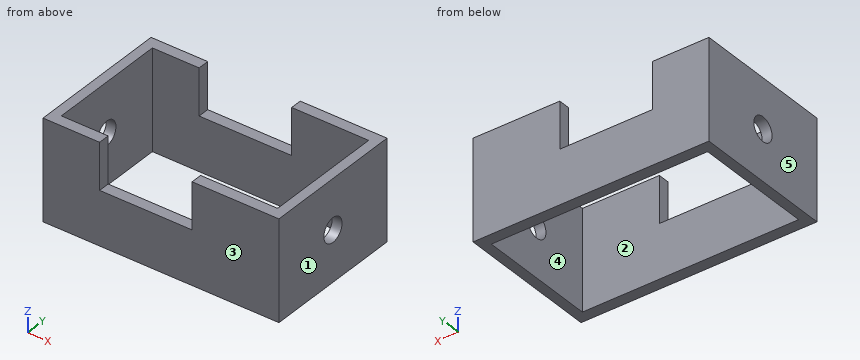
```python
from build123d import *

# Parameters (mm, degrees)
F0_W     = 170.937256
F0_H     = 103.51549
F1_DEPTH = 72.644
F2_W     = 156.719148
F2_H     = 87.184086
F3_DEPTH = 171.45
F4_W     = 67.018675
F4_H     = 33.684524
F6_DEPTH = 172.212
F7_R     = 8.715652
F8_DEPTH = 233.934


with BuildPart() as f1:
    # F0 (on Top) → F1 (new body)
    with BuildSketch(Plane.XY):
        Rectangle(F0_W, F0_H)
    extrude(amount=F1_DEPTH)

    # F2 (on face) → F3 (cut)
    with BuildSketch(Plane.XY.offset(72.644)):
        Rectangle(F2_W, F2_H)
    extrude(amount=-F3_DEPTH, mode=Mode.SUBTRACT)

    # F4 (on face) → F6 (cut)
    with BuildSketch(Plane.XZ.offset(51.757745)):
        with Locations((-10.945341, 55.801738)):
            Rectangle(F4_W, F4_H)
    extrude(amount=-F6_DEPTH, mode=Mode.SUBTRACT)

    # F7 (on face) → F8 (cut)
    with BuildSketch(Plane.YZ.offset(85.468628)):
        with Locations((0, 36.621507)):
            Circle(F7_R)
    extrude(amount=-F8_DEPTH, mode=Mode.SUBTRACT)


solid = f1.part
```
Input: part model. Units: mm. Frame: model coordinates. Face numbers are marked on the shaded views. A direction names the side the tool comes from. Round coordinates to 2 decimals unless told otherwise and drop trailing zeros. Order: outer loops, then holes, each group sorted by start corner. A loop starts at its lowest first (then second) coordinate and runs counter-clockwise, first axis right, second up. Notation, with made-up numbers: (-16, -16.5) - (17, -16.5) arc R15 ccw to (17, 9.5) - close; hole circle Ø11 at (75.25, -5). An arc over 180 degrees is marked (long way). One line per question, with ' | ' between items. Start each with the question number.
1) Cut plane C-C, the plane z = 56.5. Return the cut outline in (x, y), then the cut area to 3 significant figures.
2) Pull-direction query (Y, two-part tool) for the marked faces 3, 4 and 5; classes: +Y half, -Y half, draft (parallel to the pull), parting line (faces both ways), or undercut.
3) Set-up query: the marked faces 1 and 2. Return all of +Z, -Z, +X, -X, +Y, -Y with unobstructed straight access to the full face (end or side cutting, diameter ignored); none if empty.
4) Cut plane D-D, the plane z = 42.5. Return the cut outline in (x, y), then the cut area to 3 significant figures.
5) Ray query, probe 1 along Y at (x, z) = (71, 27); probe 2 along X at (y, z) = (-19.5, 37); probe 3 along Z at (x, y) = (-81, 0). Return the intervals inside material, ascending.
6) Cut plane B-B, the plane x = 56. Return the cut outline in (y, z), then the cut area to 3 significant figures.
7) Cut plane A-A, the plane y = 0. Return the cut outline in (x, z), then the cut area to 3 significant figures.
8) Contact query for flat-ended pins moving along their axis: P1, Ø14, axis at y = 0, z = 36.62, coming from the +X side; P2, Ø6.5, axis at x = 0.5, y = 48.5, coming from the +Z side. Output: stop coordinate, or through.
Worked out:
1) outline: (-85.47, -51.76) - (-44.45, -51.76) - (-44.45, -43.59) - (-78.36, -43.59) - (-78.36, 43.59) - (-44.45, 43.59) - (-44.45, 51.76) - (-85.47, 51.76) - close; (22.56, -51.76) - (85.47, -51.76) - (85.47, 51.76) - (22.56, 51.76) - (22.56, 43.59) - (78.36, 43.59) - (78.36, -43.59) - (22.56, -43.59) - close | area: 2,940 mm^2
2) face 3: -Y half | face 4: undercut | face 5: draft
3) face 1: +Z, -Z, +X, +Y, -Y | face 2: +Z, -Z
4) outline: (-85.47, -51.76) - (-44.45, -51.76) - (-44.45, -43.59) - (-78.36, -43.59) - (-78.36, -6.43) - (-85.47, -6.43) - close; (-85.47, 6.43) - (-78.36, 6.43) - (-78.36, 43.59) - (-44.45, 43.59) - (-44.45, 51.76) - (-85.47, 51.76) - close; (22.56, -51.76) - (85.47, -51.76) - (85.47, -6.43) - (78.36, -6.43) - (78.36, -43.59) - (22.56, -43.59) - close; (22.56, 43.59) - (78.36, 43.59) - (78.36, 6.43) - (85.47, 6.43) - (85.47, 51.76) - (22.56, 51.76) - close | area: 2,750 mm^2
5) probe 1: y = -51.76 to -43.59, 43.59 to 51.76 | probe 2: x = -85.47 to -78.36, 78.36 to 85.47 | probe 3: z = 0 to 27.91, 45.34 to 72.64
6) outline: (-51.76, 0) - (-43.59, 0) - (-43.59, 72.64) - (-51.76, 72.64) - close; (43.59, 0) - (51.76, 0) - (51.76, 72.64) - (43.59, 72.64) - close | area: 1,190 mm^2
7) outline: (-85.47, 0) - (-78.36, 0) - (-78.36, 27.91) - (-85.47, 27.91) - close; (-85.47, 45.34) - (-78.36, 45.34) - (-78.36, 72.64) - (-85.47, 72.64) - close; (78.36, 0) - (85.47, 0) - (85.47, 27.91) - (78.36, 27.91) - close; (78.36, 45.34) - (85.47, 45.34) - (85.47, 72.64) - (78.36, 72.64) - close | area: 785 mm^2
8) P1: passes through | P2: stops at z = 38.96
